Check sheet for the modelled part. Datum: model origin and axes. Units: mm. Face numbers are marked on the shaded views. A direction names the side the tool comes from. Round coordinates to 2 decimals unless told otherwise and drop trailing zeros. Write each loop counter-clockwise with the first axis right and the second up, starting at its lowest first coordinate (ties: lowest second). Pieces come first, ordered by that corner, then holes. Notation, with made-up numbers: (54, 81) - (105, 81) arc R27 ccw to (105, 100) - close; hole circle Ø8 at (63.25, 12.5). An arc over 180 degrees is marked (long way). Answer as a JSON object with one key per item and string values. Group by question number.
Item 1: Sectioned sample at A-A on z = -33. Record the boundary of the cut face in (x, y), plus the area to 3 significant figures.
Item 2: Release check for a two-part mould opening along X. For the marked faces 1, 2 and 3 record: pulls with the +X half, pulls with the -X half, needs draft (parallel to the pull), parting line crosses it, or undercut.
Item 3: Set-up check for the marked faces 4, 5, 6, 7 and 8: record each of +Z, -Z, +X, -X, +Y, -Y from which the full face is reachable in a straight line by a thin tool's end or side.
Item 4: Gauge pin test, flat ends, axial feed: P1, Ø3.5, axis at y = 5.5, z = -36.5, coming from the -X side; P2, Ø10.5, axis at x = 0, y = -6, coming from the -Z side (3 decimals); P3, Ø6, axis at x = -5, z = -19.5, coming from the +Y side; P4, Ø6, axis at y = -5, z = -9, coming from the +X side. Record the tip position at first contact, or that the pin passes through.
Item 5: Sectioned sample at D-D on y = -3.5. Record the boundary of the cut face in (x, z) (3 decimals).
Item 6: Thickness scan on line 1 (X direction, y = 5.5, z = -37.5); line 2 (X direction, y = 0.25, z = -5); line 3 (Z direction, x = 10, y = 0.5) (3 decimals). Record the ranges inside material, lowest first.
Item 7: Sectioned sample at C-C on z = 1.5. Record the boundary of the cut face in (x, y), plus the area to 3 significant figures.
Item 8: Sectioned sample at B-B on x = -12. Record the boundary of the cut face in (y, z) (3 decimals).
```python
from build123d import *

# Parameters (mm, degrees)
SKETCH2_W               = 11.9687594
SKETCH2_H               = 2.75
BOSS_EXTRUDE1_DEPTH     = 9.525
BOSS_EXTRUDE2_START     = 3.175
SKETCH2_3_W             = 11.9687594
SKETCH2_3_H             = 2.75
SKETCH2_3_W_2           = 4.572
SKETCH2_3_H_2           = 5.334
BOSS_EXTRUDE2_DEPTH     = 6.35
BOSS_EXTRUDE3_DEPTH     = 2
BOSS_EXTRUDE7_DEPTH     = 25.4
SKETCH5_W               = 9.771111266
SKETCH5_H               = 3
CUT_EXTRUDE1_DEPTH      = 78.484078326
SKETCH6_W               = 30.314979468
SKETCH6_H               = 2.000002
SKETCH6_W_2             = 22.73097918
SKETCH6_H_2             = 6.646875
CUT_EXTRUDE2_DEPTH      = 20.258872
CUT_EXTRUDE3_START      = 0.499999
SKETCH6_3_W             = 22.73097918
SKETCH6_3_H             = 2.000002
SKETCH6_3_H_2           = 4.646873
SKETCH6_3_W_2           = 0.271399
SKETCH6_3_H_3           = 3
CUT_EXTRUDE3_DEPTH      = 7.0000114
FILLET2_R               = 17.78
CUT_EXTRUDE4_DEPTH      = 48.132860149
CUT_EXTRUDE4_DEPTH_BACK = 48.132860149
SKETCH7_W               = 8.7937594
SKETCH7_H               = 20.387434944
FILLET3_R               = 2.54
SKETCH8_W               = 1.515000072
SKETCH8_H               = 2.54
BOSS_EXTRUDE8_DEPTH     = 2
FILLET4_R               = 5.08
CUT_EXTRUDE5_DEPTH      = 49.292968639


with BuildPart() as part:
    # Sketch2 → Boss-Extrude1 (new body)
    with BuildSketch(Plane.XY):
        with BuildLine():
            ThreePointArc((-9e-09, 2.75), (-3.109063455, 4.037816251), (-4.3968797, 7.1468797))
            Line((-4.3968797, 7.1468797), (-5.9843797, 7.1468797))
            Line((-5.9843797, 7.1468797), (-5.9843797, 2.75))
            Line((-5.9843797, 2.75), (-9e-09, 2.75))
        make_face()
        with BuildLine():
            Line((5.9843797, 7.1468797), (4.3968797, 7.1468797))
            ThreePointArc((4.3968797, 7.1468797), (3.109063449, 4.037816245), (-9e-09, 2.75))
            Line((-9e-09, 2.75), (5.9843797, 2.75))
            Line((5.9843797, 2.75), (5.9843797, 7.1468797))
        make_face()
        with Locations((0, 1.375)):
            Rectangle(SKETCH2_W, SKETCH2_H)
    extrude(amount=BOSS_EXTRUDE1_DEPTH)

    # Sketch2<3> → Boss-Extrude2 (add)
    with BuildSketch(Plane.XY.offset(BOSS_EXTRUDE2_START)):
        with Locations((0, 1.375)):
            Rectangle(SKETCH2_3_W, SKETCH2_3_H)
        with BuildLine():
            ThreePointArc((-9e-09, 2.75), (-3.109063455, 4.037816251), (-4.3968797, 7.1468797))
            Line((-4.3968797, 7.1468797), (-5.9843797, 7.1468797))
            Line((-5.9843797, 7.1468797), (-5.9843797, 2.75))
            Line((-5.9843797, 2.75), (-9e-09, 2.75))
        make_face()
        with BuildLine():
            Line((5.9843797, 7.1468797), (4.3968797, 7.1468797))
            ThreePointArc((4.3968797, 7.1468797), (3.109063449, 4.037816245), (-9e-09, 2.75))
            Line((-9e-09, 2.75), (5.9843797, 2.75))
            Line((5.9843797, 2.75), (5.9843797, 7.1468797))
        make_face()
        with Locations((0, -2.667)):
            Rectangle(SKETCH2_3_W_2, SKETCH2_3_H_2)
        Polygon((2.286, -5.334), (-2.286, -5.334), (-4.826, -5.334), (-4.826, -14.859), (4.826, -14.859), (4.826, -5.334), align=None)
    extrude(amount=BOSS_EXTRUDE2_DEPTH)

    # Sketch3 → Boss-Extrude3 (add)
    with BuildSketch(Plane.XZ):
        Polygon((14.9225, 9.525), (-14.9225, 9.525), (-14.9225, -22.225), (-10.85748959, -22.225), (10.85748959, -22.225), (14.9225, -22.225), align=None)
    extrude(amount=-BOSS_EXTRUDE3_DEPTH)

    # Sketch4<6> → Boss-Extrude7 (add, symmetric)
    with BuildSketch(Plane(origin=(0, 0, 0), x_dir=(0, 0, -1), z_dir=(1, 0, 0))):
        Polygon((28.087296632, 3.646875), (41.146305566, 3.646875), (41.146305566, 6.646875), (25.209889757, 6.646875), (17.740108187, 2), (22.225, 0), align=None)
    extrude(amount=BOSS_EXTRUDE7_DEPTH, both=True)

    # Sketch5 → Cut-Extrude1 (cut, through all)
    with BuildSketch(Plane(origin=(0, 37.971305566, -41.146305566), x_dir=(1, 0, 0), z_dir=(0, 0, 1))):
        Polygon((25.4, -37.971305566), (25.4, -34.324430566), (15.628888734, -34.324430566), (14.9225, -34.324430566), (14.9225, -37.971305566), align=None)
        with Locations((20.514444367, -32.824430566)):
            Rectangle(SKETCH5_W, SKETCH5_H)
        Polygon((-25.4, -34.324430566), (-25.4, -37.971305566), (-14.9225, -37.971305566), (-14.9225, -34.324430566), (-15.628888734, -34.324430566), align=None)
        with Locations((-20.514444367, -32.824430566)):
            Rectangle(SKETCH5_W, SKETCH5_H)
    extrude(amount=CUT_EXTRUDE1_DEPTH, mode=Mode.SUBTRACT)

    # Sketch6 → Cut-Extrude2 (cut)
    with BuildSketch(Plane(origin=(0, 0, -40.646306566), x_dir=(-1, 0, 0), z_dir=(0, 0, -1))):
        with Locations((0, 5.646874)):
            Rectangle(SKETCH6_W, SKETCH6_H)
        with Locations((0, 3.3234375)):
            Rectangle(SKETCH6_W_2, SKETCH6_H_2)
    extrude(amount=-CUT_EXTRUDE2_DEPTH, mode=Mode.SUBTRACT)

    # Sketch6<3> → Cut-Extrude3 (cut)
    with BuildSketch(Plane(origin=(0, 0, -40.646306566), x_dir=(-1, 0, 0), z_dir=(0, 0, -1)).offset(CUT_EXTRUDE3_START)):
        with Locations((0, 5.646874)):
            Rectangle(SKETCH6_3_W, SKETCH6_3_H)
        with Locations((0, 2.3234365)):
            Rectangle(SKETCH6_3_W, SKETCH6_3_H_2)
        with Locations((-15.493189234, 5.146875)):
            Rectangle(SKETCH6_3_W_2, SKETCH6_3_H_3)
        with Locations((15.493189234, 5.146875)):
            Rectangle(SKETCH6_3_W_2, SKETCH6_3_H_3)
    extrude(amount=-CUT_EXTRUDE3_DEPTH, mode=Mode.SUBTRACT)

    # Fillet2
    # the kernel refuses this fillet: 17.78 mm, written as the material it adds along each edge
    with BuildSketch(Plane(origin=(27.620205217, 2, -17.740108187), x_dir=(0, 0.5282208325858079, -0.8491070321357349), z_dir=(-1, 0, 0))) as fillet2_piece_1_section:
        with BuildLine():
            CenterArc((FILLET2_R * 0.285662659546, -FILLET2_R), FILLET2_R, 90, 31.885322289)
            Line((-FILLET2_R * 0.242558173039, -FILLET2_R * 0.150892967864), (0, 0))
            Line((0, 0), (FILLET2_R * 0.285662659546, 0))
        make_face()
    fillet2_piece_1 = extrude(amount=55.240410434, mode=Mode.PRIVATE)
    fillet2_piece_1 = split(fillet2_piece_1, bisect_by=Plane(origin=(15.393189234, 3.646875, -22.00929754), z_dir=(0, 1, 0)), keep=Keep.TOP, mode=Mode.PRIVATE)
    fillet2_piece_1 = split(fillet2_piece_1, bisect_by=Plane(origin=(15.628888734, 4.655865618, -22.00929754), z_dir=(-1, 0, 0)), keep=Keep.TOP, mode=Mode.PRIVATE)
    fillet2_piece_1 = split(fillet2_piece_1, bisect_by=Plane(origin=(15.157489734, 4.655865618, -22.00929754), z_dir=(1, 0, 0)), keep=Keep.TOP, mode=Mode.PRIVATE)
    add(fillet2_piece_1)
    with BuildSketch(Plane(origin=(27.620205217, 2, -17.740108187), x_dir=(0, 0.5282208325858079, -0.8491070321357349), z_dir=(-1, 0, 0))) as fillet2_piece_2_section:
        with BuildLine():
            CenterArc((FILLET2_R * 0.285662659546, -FILLET2_R), FILLET2_R, 90, 31.885322289)
            Line((-FILLET2_R * 0.242558173039, -FILLET2_R * 0.150892967864), (0, 0))
            Line((0, 0), (FILLET2_R * 0.285662659546, 0))
        make_face()
    fillet2_piece_2 = extrude(amount=55.240410434, mode=Mode.PRIVATE)
    fillet2_piece_2 = split(fillet2_piece_2, bisect_by=Plane(origin=(15.039994889, 3.646875, -20.807533434), z_dir=(0, 1, 0)), keep=Keep.TOP, mode=Mode.PRIVATE)
    fillet2_piece_2 = split(fillet2_piece_2, bisect_by=Plane(origin=(15.157489734, 3.944287392, -20.807533434), z_dir=(-1, 0, 0)), keep=Keep.TOP, mode=Mode.PRIVATE)
    fillet2_piece_2 = split(fillet2_piece_2, bisect_by=Plane(origin=(15.039994889, 4.646873, -20.807533434), z_dir=(0, -1, 0)), keep=Keep.TOP, mode=Mode.PRIVATE)
    fillet2_piece_2 = split(fillet2_piece_2, bisect_by=Plane(origin=(11.36548959, 3.944287392, -20.807533434), z_dir=(1, 0, 0)), keep=Keep.TOP, mode=Mode.PRIVATE)
    add(fillet2_piece_2)
    with BuildSketch(Plane(origin=(14.9225, 2, -17.740108187), x_dir=(0, 0.528220832585808, -0.8491070321357348), z_dir=(-1, 0, 0))) as fillet2_piece_3_section:
        with BuildLine():
            CenterArc((FILLET2_R * 0.285662659546, -FILLET2_R), FILLET2_R, 90, 31.885322289)
            Line((-FILLET2_R * 0.242558173039, -FILLET2_R * 0.150892967864), (0, 0))
            Line((0, 0), (FILLET2_R * 0.285662659546, 0))
        make_face()
    fillet2_piece_3 = extrude(amount=29.845, mode=Mode.PRIVATE)
    fillet2_piece_3 = split(fillet2_piece_3, bisect_by=Plane(origin=(13.143994801, 2.494402422, -20.387434566), z_dir=(0, 0, 1)), keep=Keep.TOP, mode=Mode.PRIVATE)
    add(fillet2_piece_3)
    with BuildSketch(Plane(origin=(27.620205217, 2, -17.740108187), x_dir=(0, 0.5282208325858079, -0.8491070321357349), z_dir=(-1, 0, 0))) as fillet2_piece_4_section:
        with BuildLine():
            CenterArc((FILLET2_R * 0.285662659546, -FILLET2_R), FILLET2_R, 90, 31.885322289)
            Line((-FILLET2_R * 0.242558173039, -FILLET2_R * 0.150892967864), (0, 0))
            Line((0, 0), (FILLET2_R * 0.285662659546, 0))
        make_face()
    fillet2_piece_4 = extrude(amount=55.240410434, mode=Mode.PRIVATE)
    fillet2_piece_4 = split(fillet2_piece_4, bisect_by=Plane(origin=(-15.628888734, 3.94428727, -20.807533615), z_dir=(1, 0, 0)), keep=Keep.TOP, mode=Mode.PRIVATE)
    fillet2_piece_4 = split(fillet2_piece_4, bisect_by=Plane(origin=(-13.143995303, 3.646875, -20.807533615), z_dir=(0, 1, 0)), keep=Keep.TOP, mode=Mode.PRIVATE)
    fillet2_piece_4 = split(fillet2_piece_4, bisect_by=Plane(origin=(-13.143995303, 4.646873, -20.807533615), z_dir=(0, -1, 0)), keep=Keep.TOP, mode=Mode.PRIVATE)
    fillet2_piece_4 = split(fillet2_piece_4, bisect_by=Plane(origin=(-11.36548959, 3.94428727, -20.807533615), z_dir=(-1, 0, 0)), keep=Keep.TOP, mode=Mode.PRIVATE)
    add(fillet2_piece_4)
    with BuildSketch(Plane(origin=(27.620205217, 2, -17.740108187), x_dir=(0, 0.5282208325858079, -0.8491070321357349), z_dir=(-1, 0, 0))) as fillet2_piece_5_section:
        with BuildLine():
            CenterArc((FILLET2_R * 0.285662659546, -FILLET2_R), FILLET2_R, 90, 31.885322289)
            Line((-FILLET2_R * 0.242558173039, -FILLET2_R * 0.150892967864), (0, 0))
            Line((0, 0), (FILLET2_R * 0.285662659546, 0))
        make_face()
    fillet2_piece_5 = extrude(amount=55.240410434, mode=Mode.PRIVATE)
    fillet2_piece_5 = split(fillet2_piece_5, bisect_by=Plane(origin=(-15.628888734, 4.655865618, -22.00929754), z_dir=(1, 0, 0)), keep=Keep.TOP, mode=Mode.PRIVATE)
    fillet2_piece_5 = split(fillet2_piece_5, bisect_by=Plane(origin=(-15.393189234, 4.655865618, -20.387434566), z_dir=(0, 0, -1)), keep=Keep.TOP, mode=Mode.PRIVATE)
    fillet2_piece_5 = split(fillet2_piece_5, bisect_by=Plane(origin=(-15.157489734, 4.655865618, -22.00929754), z_dir=(-1, 0, 0)), keep=Keep.TOP, mode=Mode.PRIVATE)
    add(fillet2_piece_5)

    # Sketch7 → Cut-Extrude4 (cut, two sides: drawn at the far end of the back side and taken through both)
    with BuildSketch(Plane(origin=(0, 2, 0), x_dir=(1, 0, 0), z_dir=(0, 1, 0)).offset(-CUT_EXTRUDE4_DEPTH_BACK)):
        with Locations((0, 10.193717472)):
            Rectangle(SKETCH7_W, SKETCH7_H)
    extrude(amount=CUT_EXTRUDE4_DEPTH + CUT_EXTRUDE4_DEPTH_BACK, mode=Mode.SUBTRACT)

    # Fillet3
    fillet3_edges = [part.edges().sort_by_distance(p)[0] for p in [
        (4.3968797, 1, 0),
        (-4.3968797, 1, 0),
    ]]
    fillet(fillet3_edges, radius=FILLET3_R)

    # Sketch8 → Boss-Extrude8 (add)
    with BuildSketch(Plane(origin=(0, 4.646873, 0), x_dir=(1, 0, 0), z_dir=(0, 1, 0))):
        with Locations((-14.399989698, 27.176306566)):
            Rectangle(SKETCH8_W, SKETCH8_H)
        with Locations((14.399989698, 27.176306566)):
            Rectangle(SKETCH8_W, SKETCH8_H)
    extrude(amount=BOSS_EXTRUDE8_DEPTH)

    # Fillet4
    fillet4_edges = [part.edges().sort_by_distance(p)[0] for p in [
        (11.36548959, 1.883268266, -20.387434566),
        (-11.36548959, 1.883268266, -20.387434566),
    ]]
    fillet(fillet4_edges, radius=FILLET4_R)

    # Sketch10 → Cut-Extrude5 (cut, through all)
    with BuildSketch(Plane(origin=(4.826, 0, 0), x_dir=(0, 0, -1), z_dir=(1, 0, 0))):
        with BuildLine():
            Line((-6.243675471, -13.842705282), (-9.525, -5.334))
            Line((-9.525, -5.334), (-9.525, -14.859))
            Line((-9.525, -14.859), (-4.7625, -14.859))
            ThreePointArc((-4.7625, -14.859), (-5.660655851, -14.580496684), (-6.243675471, -13.842705282))
        make_face()
        with BuildLine():
            ThreePointArc((-3.175, -13.2715), (-3.639967985, -14.394032015), (-4.7625, -14.859))
            Line((-4.7625, -14.859), (-3.175, -14.859))
            Line((-3.175, -14.859), (-3.175, -13.2715))
        make_face()
    extrude(amount=-CUT_EXTRUDE5_DEPTH, mode=Mode.SUBTRACT)


solid = part.part
```
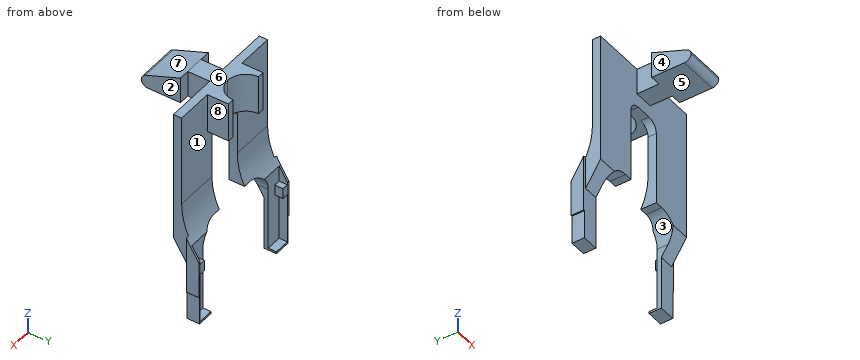
Completed:
{
 "1": {"outline": "(-15.63, 3.65) - (-11.37, 3.65) - (-11.37, 4.65) - (-15.16, 4.65) - (-15.16, 6.65) - (-15.63, 6.65) - close; (11.37, 3.65) - (15.63, 3.65) - (15.63, 6.65) - (15.16, 6.65) - (15.16, 4.65) - (11.37, 4.65) - close", "area": "10.4 mm²"},
 "2": {"face 1": "needs draft", "face 2": "pulls with the +X half", "face 3": "undercut"},
 "3": {"face 4": "+Z, -Z, -X, -Y", "face 5": "-Z, +X, -X, -Y", "face 6": "+Z, +X, -X, +Y, -Y", "face 7": "+Z, +X, -X, -Y", "face 8": "+Z, +X, +Y"},
 "4": {"P1": "x = -15.36", "P2": "z = 3.175", "P3": "y = 3.88", "P4": "through"},
 "5": {"outline": "(-2.286, 3.175) - (2.286, 3.175) - (2.286, 9.525) - (-2.286, 9.525) - close"},
 "6": {"line 1": "-15.36 to -15.16, 15.16 to 15.36", "line 2": "-14.92 to -4.4, 4.4 to 14.92", "line 3": "-22.002 to 9.525"},
 "7": {"outline": "(-14.92, 0) - (14.92, 0) - (14.92, 2) - (5.98, 2) - (5.98, 7.15) - (4.4, 7.15) arc R4.4 cw to (-4.4, 7.15) - (-5.98, 7.15) - (-5.98, 2) - (-14.92, 2) - close", "area": "90.9 mm²"},
 "8": {"outline": "(0, -22.225) - (3.647, -28.087) - (3.647, -41.146) - (6.647, -41.146) - (6.647, -40.646) - (4.647, -40.646) - (4.647, -21.995) arc R17.78 cw to (2, -12.661) - (2, 9.525) - (0, 9.525) - close"}
}
